CAD build for the part. Positions are in the model's coordinates, mm. A direction names the side the tool comes from. Give positions to 0.01 mm unless a question says otherwise; leave off trailing zeros. Write each loop counter-clockwise with the first axis right and the second up, starting at its lowest first coordinate (ties: lowest second). Pieces come first, ordered by that corner, then holes. Notation, with made-up numbers: (1.5, -13) - (10.5, -13) arc R18 cw to (10.5, 10) - close; hole circle Ø9 at (40, 59). An arc over 180 degrees is marked (long way). Answer as a JSON object with one key per item and string values.
from build123d import *

# Parameters (mm, degrees)
SKETCH_W          = 125
SKETCH_H          = 102
PAD_DEPTH         = 5.9
POCKET_DEPTH      = 7
POCKET001_DEPTH   = 7
POCKET003_DEPTH   = 6
POCKET004_DEPTH   = 6
SKETCH008_R       = 4
PAD002_DEPTH      = 4
SKETCH009_R       = 1.5
POCKET005_DEPTH   = 9
SKETCH010_R       = 6
PAD003_DEPTH      = 0.5
PAD003_DEPTH_BACK = 5.9
SKETCH011_R       = 3
PAD004_DEPTH      = 2
SKETCH012_R       = 1.5
POCKET006_DEPTH   = 8
SKETCH013_R       = 1.6
POCKET007_DEPTH   = 5.901


with BuildPart() as part:
    # Sketch → Pad (new body)
    with BuildSketch(Plane.XY):
        with Locations((62.5, 51)):
            Rectangle(SKETCH_W, SKETCH_H)
    extrude(amount=PAD_DEPTH)

    # Sketch001 (on Face3 of Pad) → Pocket (cut)
    with BuildSketch(Plane.XZ):
        Polygon((7.4, 5.9), (17.6, 5.9), (20.1, 0), (4.9, 0), align=None)
        Polygon((32.4, 5.9), (42.6, 5.9), (45.1, 0), (29.9, 0), align=None)
        Polygon((57.4, 5.9), (67.6, 5.9), (70.1, 0), (54.9, 0), align=None)
        Polygon((82.4, 5.9), (92.6, 5.9), (95.1, 0), (79.9, 0), align=None)
        Polygon((107.4, 5.9), (117.6, 5.9), (120.1, 0), (104.9, 0), align=None)
    extrude(amount=-POCKET_DEPTH, mode=Mode.SUBTRACT)

    # Sketch003 (on Face1 of Pocket) → Pocket001 (cut)
    with BuildSketch(Plane(origin=(0, 102, 0), x_dir=(-1, 0, 0), z_dir=(0, 1, 0))):
        Polygon((-117.6, 5.9), (-107.4, 5.9), (-104.9, 0), (-120.1, 0), align=None)
        Polygon((-92.6, 5.9), (-82.4, 5.9), (-79.9, 0), (-95.1, 0), align=None)
        Polygon((-67.6, 5.9), (-57.4, 5.9), (-54.9, 0), (-70.1, 0), align=None)
        Polygon((-42.6, 5.9), (-32.4, 5.9), (-29.9, 0), (-45.1, 0), align=None)
        Polygon((-17.4, 5.9), (-7.6, 5.9), (-4.9, 0), (-20.1, 0), align=None)
    extrude(amount=-POCKET001_DEPTH, mode=Mode.SUBTRACT)

    # Sketch006 → Pocket003 (cut)
    with BuildSketch(Plane(origin=(0, 0, 0), x_dir=(1, 0, 0), z_dir=(0, 0, -1))):
        Polygon((15.5, -17), (109.5, -17), (62.5, -47), align=None)
        Polygon((15.5, -86), (109.5, -86), (62.5, -56), align=None)
    extrude(amount=-POCKET003_DEPTH, mode=Mode.SUBTRACT)

    # Sketch007 (on Face4 of Pocket003) → Pocket004 (cut)
    with BuildSketch(Plane.XY.offset(5.9)):
        Polygon((15.5, 81), (15.5, 21), (58.5, 51), align=None)
        Polygon((109.5, 81), (109.5, 21), (66.5, 51), align=None)
    extrude(amount=-POCKET004_DEPTH, mode=Mode.SUBTRACT)

    # Sketch008 (on Face4 of Pocket004) → Pad002 (join)
    with BuildSketch(Plane.XY.offset(5.9)):
        with Locations((11.5, 89)):
            Circle(SKETCH008_R)
        with Locations((113.5, 89)):
            Circle(SKETCH008_R)
        with Locations((11.5, 13)):
            Circle(SKETCH008_R)
        with Locations((113.5, 13)):
            Circle(SKETCH008_R)
    extrude(amount=PAD002_DEPTH)

    # Sketch009 (on Face65 of Pad002) → Pocket005 (cut)
    with BuildSketch(Plane.XY.offset(9.9)):
        with Locations((11.5, 13)):
            Circle(SKETCH009_R)
        with Locations((11.5, 89)):
            Circle(SKETCH009_R)
        with Locations((113.5, 89)):
            Circle(SKETCH009_R)
        with Locations((113.5, 13)):
            Circle(SKETCH009_R)
    extrude(amount=-POCKET005_DEPTH, mode=Mode.SUBTRACT)

    # Sketch010 (on Face4 of Pocket005) → Pad003 (join, two sides)
    with BuildSketch(Plane.XY.offset(5.9)) as pad003_sk:
        with Locations((33.5, 75.5)):
            Circle(SKETCH010_R)
        with Locations((91.5, 75.5)):
            Circle(SKETCH010_R)
        with Locations((33.5, 26.5)):
            Circle(SKETCH010_R)
        with Locations((91.5, 26.5)):
            Circle(SKETCH010_R)
    extrude(amount=PAD003_DEPTH)
    extrude(pad003_sk.sketch, amount=-PAD003_DEPTH_BACK)

    # Sketch011 (on Face4 of Pad003) → Pad004 (join)
    with BuildSketch(Plane.XY.offset(5.9)):
        with Locations((33.5, 75.5)):
            Circle(SKETCH011_R)
        with Locations((91.5, 75.5)):
            Circle(SKETCH011_R)
        with Locations((33.5, 26.5)):
            Circle(SKETCH011_R)
        with Locations((91.5, 26.5)):
            Circle(SKETCH011_R)
    extrude(amount=PAD004_DEPTH)

    # Sketch012 (on Face108 of Pad004) → Pocket006 (cut)
    with BuildSketch(Plane.XY.offset(7.9)):
        with Locations((91.5, 75.5)):
            Circle(SKETCH012_R)
        with Locations((91.5, 26.5)):
            Circle(SKETCH012_R)
        with Locations((33.5, 26.5)):
            Circle(SKETCH012_R)
        with Locations((33.5, 75.5)):
            Circle(SKETCH012_R)
    extrude(amount=-POCKET006_DEPTH, mode=Mode.SUBTRACT)

    # Sketch013 (on Face4 of Pocket006) → Pocket007 (cut, through all)
    with BuildSketch(Plane.XY.offset(5.9)):
        with Locations((25, 3.5)):
            Circle(SKETCH013_R)
        with Locations((50, 3.5)):
            Circle(SKETCH013_R)
        with Locations((75, 3.5)):
            Circle(SKETCH013_R)
        with Locations((100, 3.5)):
            Circle(SKETCH013_R)
        with Locations((25, 98.5)):
            Circle(SKETCH013_R)
        with Locations((50, 98.5)):
            Circle(SKETCH013_R)
        with Locations((75, 98.5)):
            Circle(SKETCH013_R)
        with Locations((100, 98.5)):
            Circle(SKETCH013_R)
    extrude(amount=-POCKET007_DEPTH, mode=Mode.SUBTRACT)


solid = part.part
(1) 3-axis set-ups, long thin cutter, end or side, ignore diameter. For faces 3 (the face through (106.168, 98.549, 2.991)), 4 (the face through (6.133, 3.451, 2.909)), 5 (the face through (11, 13, 0.9)), 6 (the face through (45.18, 60.293, 2.991)): which of +Z, -Z, +X, -X, +Y, -Y reach the whole face in a straight line?
Answer key:
{"face 3": "-Z, +Y", "face 4": "-Z, -Y", "face 5": "+Z", "face 6": "+Z, -Z"}
(2) Saw through at D-D, the plane y = 13. Give the cut face in (x, z).
Answer key:
{"outline": "(0, 0) - (125, 0) - (125, 5.9) - (117.5, 5.9) - (117.5, 9.9) - (115, 9.9) - (115, 0.9) - (112, 0.9) - (112, 9.9) - (109.5, 9.9) - (109.5, 5.9) - (15.5, 5.9) - (15.5, 9.9) - (13, 9.9) - (13, 0.9) - (10, 0.9) - (10, 9.9) - (7.5, 9.9) - (7.5, 5.9) - (0, 5.9) - close"}
(3) Saw through at B-B, the plane x = 100. Give the cut face in (y, z), and give its area (3 significant figures).
Answer key:
{"outline": "(0, 0) - (1.9, 0) - (1.9, 5.9) - (0, 5.9) - close; (5.1, 0) - (17, 0) - (17, 5.9) - (5.1, 5.9) - close; (23.06, 0) - (27.63, 0) - (27.63, 5.9) - (23.06, 5.9) - close; (74.37, 0) - (79.94, 0) - (79.94, 5.9) - (74.37, 5.9) - close; (86, 0) - (96.9, 0) - (96.9, 5.9) - (86, 5.9) - close; (100.1, 0) - (102, 0) - (102, 5.9) - (100.1, 5.9) - close", "area": "217 mm²"}
(4) Probe L1, parallel to Y at x = 11.5, z = 7.25; L2, parallel to X at y = 75.5, z = 2.25; L3, parallel to Y at x = 64, z = 2.25. List the from-to ranges inside material, lowest first. Write a range as [from, to].
Answer key:
{"L1": "y = [9, 11.5], [14.5, 17], [85, 87.5], [90.5, 93]", "L2": "x = [0, 15.5], [23.38, 32], [35, 39.5], [85.5, 90], [93, 101.62], [109.5, 125]", "L3": "y = [7, 17], [46.04, 56.96], [86, 95]"}
(5) Saw through at A-A, the plane y = 49.5. Give the cut face in (x, z), and give its area (3 significant figures).
Answer key:
{"outline": "(0, 0) - (15.5, 0) - (15.5, 5.9) - (0, 5.9) - close; (56.35, 0) - (68.65, 0) - (68.65, 5.9) - (56.35, 5.9) - close; (109.5, 0) - (125, 0) - (125, 5.9) - (109.5, 5.9) - close", "area": "255 mm²"}
(6) Pull direction X, two halves, no side cores. Call faces 1 (the face through (76.526, 98.981, 2.991)), 2 (the face through (3, 0, 3)): pulls with the +X half, pulls with the -X half, needs draft (parallel to the pull), parting line crosses it, or undercut.
Answer key:
{"face 1": "undercut", "face 2": "needs draft"}
(7) Flat gauge pins, fed straight in: P1, Ø5, axis at x = 25.5, z = 3.5, coming from the -Y side; P2, Ø20.5, axis at x = 50, y = 50, coming from the +Z side; P3, Ø1.8, axis at x = 63.5, z = 3, coming from the +Y side; P4, Ø2.5, axis at x = 25, y = 3.5, coming from the +Z side. Where does each tip first touch, or does it go through?
Answer key:
{"P1": "stops at y = 0", "P2": "stops at z = 5.9", "P3": "stops at y = 95", "P4": "passes through"}
(8) Saw through at C-C, the plane x = 113.5. Give the cut face in (y, z), and give its area (3 significant figures).
Answer key:
{"outline": "(7, 0) - (95, 0) - (95, 5.9) - (93, 5.9) - (93, 9.9) - (90.5, 9.9) - (90.5, 0.9) - (87.5, 0.9) - (87.5, 9.9) - (85, 9.9) - (85, 5.9) - (17, 5.9) - (17, 9.9) - (14.5, 9.9) - (14.5, 0.9) - (11.5, 0.9) - (11.5, 9.9) - (9, 9.9) - (9, 5.9) - (7, 5.9) - close", "area": "529 mm²"}
